```python
from build123d import *

# Parameters (mm, degrees)
PAD_DEPTH       = 16
POCKET_DEPTH    = 1
POCKET001_DEPTH = 1


with BuildPart() as part:
    # Sketch → Pad (new body)
    with BuildSketch(Plane.XY):
        Polygon((0, 413.879036), (0, 500), (470, 500), (470, 0), (0, 0), align=None)
    extrude(amount=-PAD_DEPTH)

    # Sketch002 (on Face7 of Pad) → Pocket (cut)
    with BuildSketch(Plane(origin=(0, 0, -16), x_dir=(1, 0, 0), z_dir=(0, 0, -1))):
        Polygon((0, 0), (0, -71.973152), (470, 0), align=None)
    extrude(amount=-POCKET_DEPTH, mode=Mode.SUBTRACT)

    # Sketch003 (on Face4 of Pocket) → Pocket001 (cut)
    with BuildSketch(Plane.XY):
        Polygon((72.935243, 306.382776), (13.373917, 268.440454), (72.935243, 230.498132), (72.935243, 255.613788), (146.197296, 255.613788), (146.197296, 281.26712), (72.935243, 281.26712), align=None)
    extrude(amount=-POCKET001_DEPTH, mode=Mode.SUBTRACT)


solid = part.part
```
CAD build for the part. Positions are in the model's coordinates, mm. A direction names the side the tool comes from. Round coordinates to 2 decimals unless told otherwise and drop trailing zeros.
Item 1: Mould opens along X. For faces 3 (the face through (42.738, 249.735, -0.493)), 4 (the face through (179, 27, -15)), 5 (the face through (0, 253, -8)), 6 (the face through (43.572, 287.677, -0.493)) say: pulls with the +X half, pulls with the -X half, needs draft (parallel to the pull), parting line crosses it, or undercut.
Item 2: Tool access for faces 1 (the face through (470, 253, -8)), 2 (the face through (231.71, 36.49, -15.51)): list every direction of +Z, -Z, +X, -X, +Y, -Y with a clear straight run to the whole face (end or side of a thin tool).
Item 3: Probe line 1 along Z through (x, y) = (26.5, 57). List the from-to ranges inside material, lowest first.
Reported:
1. face 3: undercut
1. face 4: needs draft
1. face 5: pulls with the -X half
1. face 6: undercut
2. face 1: +Z, -Z, +X, +Y, -Y
2. face 2: -Z, -X, -Y
3. line 1: z = -15 to 0
